Model file for the job. Use its own axes, mm. Round coordinates to 2 decimals unless told otherwise and drop trailing zeros. Order: outer loops, then holes, each group sorted by start corner. A loop starts at its lowest first (then second) coordinate and runs counter-clockwise, first axis right, second up. Notation, with made-up numbers: M 16.5,89 L 64.5,89 A14 cw 64.5,115 Z; hole C -7,64 d11. An arc over 180 degrees is marked long. Return JSON: item names as keys, results as strings. Group by question number.
Item 1: Pin check, flat tips, straight feed: pin 1 Ø3 at (x, y) = (20, -32) entering from +Z; pin 2 Ø1.5 at (x, z) = (-11, 6) entering from -Y; pin 3 Ø3 at (x, z) = (5.5, 8) entering from -Y; pin 4 Ø1.5 at (x, z) = (-29, 7.5) entering from -Y. Stop position of each tip, or through.
Item 2: Slice it at C-C on y = -46.99. Write the cut outline in (x, z).
Item 3: Slice it at B-B on y = 16.5. Write the cut outline in (x, z), then the cut area to 3 significant figures.
Item 4: Slice it at A-A on x = 0. Write the cut outline in (y, z), then the cut area to 3 significant figures.
Item 5: Pull direction X, two halves, no side cores. Call faces 1 (the face through (47.69, 15.02, 4.93)), 2 (the face through (-13.1, -26.18, 4.93)), 3 (the face through (-23, 12, 0)): pulls with the +X half, pulls with the -X half, needs draft (parallel to the pull), parting line crosses it, or undercut.
Item 6: Probe line 1 along Y through (x, z) = (-41, 5); line 2 along X through (y, z) = (-41, 6); line 3 along Y through (x, z) = (0, 5). List the from-to ranges inside material, lowest first.
from build123d import *

# Parameters (mm, degrees)
SKETCH1_R           = 50
SKETCH1_R_2         = 25
BOSS_EXTRUDE1_DEPTH = 10
SKETCH3_R           = 8
CUT_EXTRUDE1_DEPTH  = 20
SKETCH4_R           = 1.5
CUT_EXTRUDE2_DEPTH  = 30


with BuildPart() as part:
    # Sketch1 → Boss-Extrude1 (new body)
    with BuildSketch(Plane.XY):
        Circle(SKETCH1_R)
        Circle(SKETCH1_R_2, mode=Mode.SUBTRACT)
    extrude(amount=BOSS_EXTRUDE1_DEPTH)

    # Sketch3 → Cut-Extrude1 (cut)
    with BuildSketch(Plane(origin=(0, 0, 0), x_dir=(-1, 0, 0), z_dir=(0, 0, -1))):
        with Locations((-14.146357726, 34.109474384)):
            Circle(SKETCH3_R)
        with Locations((14.116055163, 34.122026117)):
            Circle(SKETCH3_R)
        with Locations((34.109474384, 14.146357726)):
            Circle(SKETCH3_R)
        with Locations((34.122026117, -14.116055163)):
            Circle(SKETCH3_R)
        with Locations((14.146357726, -34.109474384)):
            Circle(SKETCH3_R)
        with Locations((-14.116055163, -34.122026117)):
            Circle(SKETCH3_R)
        with Locations((-34.109474384, -14.146357726)):
            Circle(SKETCH3_R)
        with Locations((-34.122026117, 14.116055163)):
            Circle(SKETCH3_R)
    extrude(amount=-CUT_EXTRUDE1_DEPTH, mode=Mode.SUBTRACT)

    # Sketch4 → Cut-Extrude2 (cut)
    with BuildSketch(Plane(origin=(0, 0, 0), x_dir=(-1, 0, 0), z_dir=(0, 0, -1))):
        with Locations((0, 46.99)):
            Circle(SKETCH4_R)
        with Locations((46.99, 0)):
            Circle(SKETCH4_R)
        with Locations((0, -46.99)):
            Circle(SKETCH4_R)
        with Locations((-46.99, 0)):
            Circle(SKETCH4_R)
    extrude(amount=-CUT_EXTRUDE2_DEPTH, mode=Mode.SUBTRACT)


solid = part.part
Output values:
{
 "1": {"pin 1": "through", "pin 2": "y = -48.94", "pin 3": "y = -49.84", "pin 4": "y = -41.25"},
 "2": {"outline": "M -17.09,0 L -1.5,0 L -1.5,10 L -17.09,10 Z; M 1.5,0 L 17.09,0 L 17.09,10 L 1.5,10 Z"},
 "3": {"outline": "M -47.2,0 L -41.76,0 L -41.76,10 L -47.2,10 Z; M -26.46,0 L -18.78,0 L -18.78,10 L -26.46,10 Z; M 18.78,0 L 26.49,0 L 26.49,10 L 18.78,10 Z; M 41.76,0 L 47.2,0 L 47.2,10 L 41.76,10 Z", "area": "263 mm²"},
 "4": {"outline": "M -50,0 L -48.49,0 L -48.49,10 L -50,10 Z; M -45.49,0 L -25,0 L -25,10 L -45.49,10 Z; M 25,0 L 45.49,0 L 45.49,10 L 25,10 Z; M 48.49,0 L 50,0 L 50,10 L 48.49,10 Z", "area": "440 mm²"},
 "5": {"face 1": "parting line crosses it", "face 2": "undercut", "face 3": "needs draft"},
 "6": {"line 1": "-28.62 to -18.2, -10.03 to 10.08, 18.21 to 28.62", "line 2": "-28.62 to -18.21, -10.08 to 10.03, 18.2 to 28.62", "line 3": "-50 to -48.49, -45.49 to -25, 25 to 45.49, 48.49 to 50"}
}
